The listing builds one solid part. Answer for the finished solid, in the listing's coordinates (mm). A direction names the side the tool comes from. Give positions to 0.01 mm unless a question says otherwise; leave off trailing zeros. Order: outer loops, then holes, each group sorted by start corner. A loop starts at its lowest first (then second) coordinate and runs counter-clockwise, first axis right, second up. Notation, with made-up numbers: (79.25, -35) - (99.25, -35) arc R34 cw to (99.25, 0) - close; hole circle Ø7 at (-31, 56.5). An arc over 180 degrees is marked (long way). Answer in a Markdown table with one row per item. Add a question column.
Autodesk Inventor part; units mm, degrees
ref_plane "YZ Plane" through (0, 0, 0) normal (1, 0, 0) x (0, 1, 0)
ref_plane "XZ Plane" through (0, 0, 0) normal (0, 1, 0) x (-1, 0, 0)
ref_plane "XY Plane" through (0, 0, 0) normal (0, 0, 1) x (1, 0, 0)
sketch "Sketch1" plane through (0, 0, 0) normal (0, 1, 0) x (-1, 0, 0)
  line L0 (20, 20) -> (20, -20)
  line L1 (20, -20) -> (-20, -20)
  line L2 (-20, -20) -> (-20, 20)
  line L3 (-20, 20) -> (20, 20)
  line L4 (-15, 15) -> (-15, -15) construction
  line L5 (-15, -15) -> (15, -15) construction
  line L6 (15, -15) -> (15, 15) construction
  line L7 (15, 15) -> (-15, 15) construction
  circle A0 centre (15, 15) radius 3.05
  circle A1 centre (15, -15) radius 3.05
  circle A2 centre (-15, -15) radius 3.05
  circle A3 centre (-15, 15) radius 3.05
  line L8 (0, 0) -> (-18.5703, 0) construction
  line L9 (0, 0) -> (0, 25.6262) construction
  line L10 (0, 0) -> (-18.05, 0) construction
  line L11 (8, 2.3333) -> (-8, 2.3333)
  line L12 (-8.5, 1.8333) -> (-8.5, 1.8333)
  line L13 (8.5, 1.8333) -> (8.5, 1.8333)
  line L14 (8.5, 2.3333) -> (-8.5, 3.0056) construction
  line L15 (-8.5, 2.3333) -> (8.5, 3.0548) construction
  arc A4 (8.5, 1.8333) -> (8, 2.3333) centre (8, 1.8333) ccw
  arc A5 (8, 1.3333) -> (8.5, 1.8333) centre (8, 1.8333) ccw
  arc A6 (-8.5, 1.8333) -> (-8, 1.3333) centre (-8, 1.8333) ccw
  arc A7 (-8, 2.3333) -> (-8.5, 1.8333) centre (-8, 1.8333) ccw
  line L16 (-8.5, -1.8333) -> (-8.5, -1.8333)
  line L17 (-8, -2.3333) -> (8, -2.3333)
  line L18 (8.5, -1.8333) -> (8.5, -1.8333)
  line L19 (8.5, -0.691) -> (-8.5, -2.3333) construction
  line L20 (-8.5, -0.6827) -> (8.5, -2.3333) construction
  arc A8 (8.5, -1.8333) -> (8.0002, -1.3333) centre (8, -1.8333) ccw
  arc A9 (8, -2.3333) -> (8.5, -1.8333) centre (8, -1.8333) ccw
  arc A10 (-8.5, -1.8333) -> (-8, -2.3333) centre (-8, -1.8333) ccw
  arc A11 (-8, -1.3333) -> (-8.5, -1.8333) centre (-8, -1.8333) ccw
  line L21 (8, 1.3333) -> (7, 1.3333)
  line L22 (7, 1.3333) -> (7, -1.3333)
  line L23 (7, -1.3333) -> (8.0002, -1.3333)
  line L24 (-8, 1.3333) -> (-7, 1.3333)
  line L25 (-7, 1.3333) -> (-7, -1.3333)
  line L26 (-7, -1.3333) -> (-8, -1.3333)
  point P0 (0, -12.01)
  point P1 (-0.3001, 2.6813)
  point P2 (0, 2.694)
  point P3 (0.0215, -1.5101)
  point P4 (0, -1.508)
  point P5 (0, -1.5122)
  dimension "d0" = 40
  dimension "d1" = 40
  dimension "d2" = 30
  dimension "d53" = 20
  dimension "d114" = 17
  dimension "d117" = 0.5
  dimension "d140" = 17
  dimension "d142" = 0.5
  dimension "d146" = 14
  dimension "d147" = 7
  dimension "d150" = 1.3333
  dimension "d151" = 1.3333
  dimension "d152" = 2.3333
  dimension "d153" = 2.3333
extrude "Extrusion15" add sketch "Sketch1" along normal blind 5
sketch "Sketch11" plane through (0, 0, 0) normal (0, -1, 0) x (1, 0, 0)
  line L0 (-11, -7.5) -> (11, -7.5)
  line L1 (12.5, -6) -> (12.5, 6)
  line L2 (11, 7.5) -> (-11, 7.5)
  line L3 (-12.5, 6) -> (-12.5, -6)
  line L4 (-12.5, -7.5) -> (12.5, 7.5) construction
  line L5 (12.5, -7.5) -> (-12.5, 7.5) construction
  arc A0 (-11, 7.5) -> (-12.5, 6) centre (-11, 6) ccw
  arc A1 (-12.5, -6) -> (-11, -7.5) centre (-11, -6) ccw
  arc A2 (11, -7.5) -> (12.5, -6) centre (11, -6) ccw
  arc A3 (12.5, 6) -> (11, 7.5) centre (11, 6) ccw
  point P0 (0, 0)
  dimension "d154" = 15
  dimension "d155" = 25
  dimension "d156" = 1.5
extrude "Extrusion16" cut sketch "Sketch11" against normal blind 3
sketch "Sketch14" plane through (0, 0, 0) normal (0, -1, 0) x (1, 0, 0)
  arc A0 (-12.5, -6) -> (-11, -7.5) centre (-11, -6) ccw
  line L0 (-12.5, -6) -> (-12.5, 6)
  arc A1 (-11, 7.5) -> (-12.5, 6) centre (-11, 6) ccw
  line L1 (-11, 7.5) -> (11, 7.5)
  arc A2 (12.5, 6) -> (11, 7.5) centre (11, 6) ccw
  line L2 (12.5, 6) -> (12.5, -6)
  arc A3 (11, -7.5) -> (12.5, -6) centre (11, -6) ccw
  line L3 (11, -7.5) -> (-11, -7.5)
  circle A4 centre (15, 15) radius 3.05
  circle A5 centre (15, -15) radius 3.05
  circle A6 centre (-15, -15) radius 3.05
  circle A7 centre (-15, 15) radius 3.05
  line L4 (-20, 20) -> (-20, -20)
  line L5 (-20, -20) -> (20, -20)
  line L6 (20, -20) -> (20, 20)
  line L7 (20, 20) -> (-20, 20)
  point P0 (0, 0)
extrude "Extrusion17" add sketch "Sketch14" along normal blind 3
sketch "Sketch12" plane through (20, 0, 20) normal (1, 0, 0) x (0, 0, -1)
  line L0 (40, 5) -> (40, -3)
  line L1 (0, 5) -> (40, 5)
  line L2 (0, 5) -> (0, -3)
  line L3 (40, -3) -> (0, -3)
  point P0 (20, 0)
  point P1 (5, 1)
  point P2 (35, 1)
  dimension "d163" = 5
  dimension "d164" = 5
  dimension "d165" = 4
  dimension "d166" = 4
hole "Hole1" at (20, 1, 15) at (20, 1, -15) direction (-1, 0, 0) diameter 2.013 depth 5 tip angle 118
sketch "Sketch13" plane through (-20, 0, -20) normal (-1, 0, 0) x (0, 0, 1)
  line L0 (40, -3) -> (40, 5)
  line L1 (0, 5) -> (40, 5)
  line L2 (0, 5) -> (0, -3)
  circle A0 centre (35, 1) radius 1.0065
  circle A1 centre (5, 1) radius 1.0065
  line L3 (40, -3) -> (0, -3)
  point P0 (20, 0)
  point P1 (33.9935, 1)
  point P2 (3.9935, 1)
hole "Hole2" at (-20, 1, 15) at (-20, 1, -15) direction (1, 0, 0) diameter 2.013 depth 5 tip angle 118
equation "\"d1\" = d0"
properties part number "HolderStart"
(1) Find section A-A, the plane y = -0.5. Write down the section's boundary in (x, z), plus the area to 3 significant figures.
(2) The mould has two halves that part along X. Classify faces 4 (the face through (20, 1, 0)), 5 (the face through (-18.925, 0.956, 13.994)), 6 (the face through (14.799, 1.056, -11.957)): +X half, -X half, draft (parallel to the pull), parting line (faces both ways), or undercut.
(3) For faces 1 (the face through (8.5, 4, -1.8)), 2 (the face through (-12.07, 0.04, 7.05)), 3 (the face through (0, 1, -20)), determine the directions among +Z, -Z, +X, -X, +Y, -Y from which every point of the face is accessible in a straight line to the end or side of a thin tool.
(4) Each of these flat-tipped pins is pushed along its axis until it touches: P1, Ø10, axis at x = -4.5, z = -1.5, coming from the +Y side; P2, Ø1.2, axis at y = 1, z = -15, coming from the +X side; P3, Ø4.5, axis at x = -4.5, z = -3.5, coming from the -Y side. Where does it stop, or does it pass through?
(5) Find section D-D, the plane y = 4.25. Write down the section's boundary in (x, z), plus the area to 3 significant figures.
(6) Find section C-C, the plane z = -3.5. Write down the section's boundary in (x, y), plus the area to 3 significant figures.
(7) Find section B-B, the plane x = 3. Write down the section's boundary in (y, z), plus the area to 3 significant figures.
(8) Straight lines are drawn through the part: line 1 (Z direction, x = 15, y = 0.75); line 2 (Z direction, x = -18.85, y = 1). For each, find the intervals that lie inside material, in ascending order.
Answer key:
| question | item | result |
|---|---|---|
| 1 | outline | (-20, -20) - (20, -20) - (20, 20) - (-20, 20) - close; hole circle Ø6.1 at (-15, -15); hole circle Ø6.1 at (-15, 15); hole (-12.5, -6) arc R1.5 ccw to (-11, -7.5) - (11, -7.5) arc R1.5 ccw to (12.5, -6) - (12.5, 6) arc R1.5 ccw to (11, 7.5) - (-11, 7.5) arc R1.5 ccw to (-12.5, 6) - close; hole circle Ø6.1 at (15, -15); hole circle Ø6.1 at (15, 15) |
| 1 | area | 1,110 mm² |
| 2 | face 4 | +X half |
| 2 | face 5 | draft |
| 2 | face 6 | undercut |
| 3 | face 1 | +Y, -Y |
| 3 | face 2 | -Y |
| 3 | face 3 | -Z, +X, -X, +Y, -Y |
| 4 | P1 | y = 5 |
| 4 | P2 | x = 12.01 |
| 4 | P3 | y = 3 |
| 5 | outline | (-20, -20) - (20, -20) - (20, 20) - (-20, 20) - close; hole circle Ø6.1 at (-15, -15); hole circle Ø6.1 at (-15, 15); hole (-8, -2.33) - (8, -2.33) arc R0.5 ccw to (8, -1.33) - (7, -1.33) - (7, 1.33) - (8, 1.33) arc R0.5 ccw to (8, 2.33) - (-8, 2.33) arc R0.5 ccw to (-8, 1.33) - (-7, 1.33) - (-7, -1.33) - (-8, -1.33) arc R0.5 ccw to start; hole circle Ø6.1 at (15, -15); hole circle Ø6.1 at (15, 15) |
| 5 | area | 1,410 mm² |
| 6 | outline | (-20, -3) - (-12.5, -3) - (-12.5, 3) - (12.5, 3) - (12.5, -3) - (20, -3) - (20, 5) - (-20, 5) - close |
| 6 | area | 170 mm² |
| 7 | outline | (-3, -20) - (5, -20) - (5, -2.33) - (3, -2.33) - (3, -7.5) - (-3, -7.5) - close; (-3, 7.5) - (3, 7.5) - (3, 2.33) - (5, 2.33) - (5, 20) - (-3, 20) - close |
| 7 | area | 221 mm² |
| 8 | line 1 | -20 to -18.05, -11.95 to 11.95, 18.05 to 20 |
| 8 | line 2 | -20 to -16.01, -13.99 to 13.99, 16.01 to 20 |
